The listing builds one solid part. Answer for the finished solid, in the listing's coordinates (mm). Face numbers are marked on the shaded views. A direction names the side the tool comes from. Coordinates: 2 decimals unless noted, no trailing zeros. Order: outer loops, then holes, each group sorted by start corner. A loop starts at its lowest first (then second) coordinate and runs counter-clockwise, first axis right, second up. Notation, with made-up numbers: (21.5, 64.25) - (35.5, 64.25) arc R11 ccw to (35.5, 81.25) - close; hole circle Ø3 at (30, 3.25). An arc over 180 degrees is marked (long way). Use one line per item in the form item = value. Start each with the question number.
Item 1: Section B-B, the plane z = 0 is taken. Write down the section's boundary in (x, y), and give its area (3 significant figures).
Item 2: Consider line 1 along X through (y, z) = (2.5, 0); line 2 along X through (y, z) = (5, 0); line 3 along Y through (x, z) = (7.5, 4). Determine where each line is inside the solid, lowest interval first. Write a range as [from, to].
Item 3: Each of these flat-tipped pins is pushed along its axis until it touches: pin 1 Ø4 at (y, z) = (17, -0.5) entering from -X; pin 2 Ø10 at (x, y) = (-20.5, 13) entering from +Z; pin 3 Ø8 at (y, z) = (28, 12.5) entering from -X. Where does it stop, or does it pass through?
Item 4: Section C-C, the plane y = 34.5 is taken. Write down the section's boundary in (x, z), and give its area (3 significant figures).
Item 5: A tool of negligible diameter and unlimited length cuts with its end or side. For the marked faces 1, 2 and 3, from which of +Z, -Z, +X, -X, +Y, -Y can it reach the whole face along a straight path? Write none if from no direction.
Item 6: Section A-A, the plane x = 0 is taken. Write down the section's boundary in (y, z).
Item 7: Section D-D, the plane y = 10.5 is taken. Write down the section's boundary in (x, z).
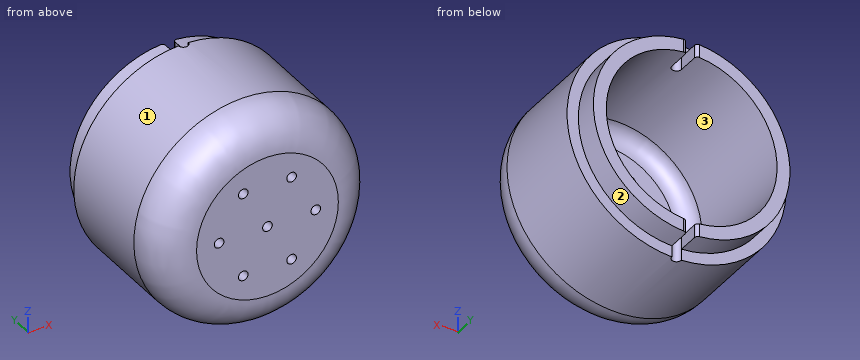
from build123d import *

# Parameters (mm, degrees)
ENL_V_MAT_EXTRU_1_REACH = 66.174
ESQUISSE2_R             = 1.5
ENL_V_MAT_EXTRU_2_DEPTH = 91.720725306
CONG_1_R                = 12
CONG_2_R                = 5
CONG_3_R                = 1


with BuildPart() as part:
    # Esquisse1 → Révolution1 (revolve)
    with BuildSketch(Plane(origin=(0, 0, 0), x_dir=(0, 0, -1), z_dir=(1, 0, 0)), mode=Mode.PRIVATE) as r_volution1_sk:
        Polygon((26.5, 49.5), (26.5, 7), (0, 7), (0, 0), (34, 0), (34, 42), (30.5, 42), (30.5, 49.5), align=None)
    revolve(r_volution1_sk.sketch.rotate(Axis((0, 7, 0), (0, -1, 0)), 180), axis=Axis((0, 7, 0), (0, -1, 0)))

    # Esquisse2 → Enlèv. mat.-Extru.1 (cut, up to next)
    with BuildSketch(Plane(origin=(0, 7, 0), x_dir=(1, 0, 0), z_dir=(0, 1, 0)), mode=Mode.PRIVATE) as enl_v_mat_extru_1_sk1:
        with Locations(Location((0, 0, 0), (0, 0, 270))):
            Circle(ESQUISSE2_R)
    enl_v_mat_extru_1_tool1 = extrude(enl_v_mat_extru_1_sk1.sketch, amount=-ENL_V_MAT_EXTRU_1_REACH, mode=Mode.PRIVATE) & part.part
    # Esquisse2 → Enlèv. mat.-Extru.1 (cut, up to next)
    with BuildSketch(Plane(origin=(0, 7, 0), x_dir=(1, 0, 0), z_dir=(0, 1, 0)), mode=Mode.PRIVATE) as enl_v_mat_extru_1_sk2:
        with Locations(Location((15, 0, 0), (0, 0, 270))):
            Circle(ESQUISSE2_R)
    enl_v_mat_extru_1_tool2 = extrude(enl_v_mat_extru_1_sk2.sketch, amount=-ENL_V_MAT_EXTRU_1_REACH, mode=Mode.PRIVATE) & part.part
    # Esquisse2 → Enlèv. mat.-Extru.1 (cut, up to next)
    with BuildSketch(Plane(origin=(0, 7, 0), x_dir=(1, 0, 0), z_dir=(0, 1, 0)), mode=Mode.PRIVATE) as enl_v_mat_extru_1_sk3:
        with Locations(Location((7.5, -12.990381057, 0), (0, 0, 270))):
            Circle(ESQUISSE2_R)
    enl_v_mat_extru_1_tool3 = extrude(enl_v_mat_extru_1_sk3.sketch, amount=-ENL_V_MAT_EXTRU_1_REACH, mode=Mode.PRIVATE) & part.part
    # Esquisse2 → Enlèv. mat.-Extru.1 (cut, up to next)
    with BuildSketch(Plane(origin=(0, 7, 0), x_dir=(1, 0, 0), z_dir=(0, 1, 0)), mode=Mode.PRIVATE) as enl_v_mat_extru_1_sk4:
        with Locations(Location((-7.5, -12.990381057, 0), (0, 0, 270))):
            Circle(ESQUISSE2_R)
    enl_v_mat_extru_1_tool4 = extrude(enl_v_mat_extru_1_sk4.sketch, amount=-ENL_V_MAT_EXTRU_1_REACH, mode=Mode.PRIVATE) & part.part
    # Esquisse2 → Enlèv. mat.-Extru.1 (cut, up to next)
    with BuildSketch(Plane(origin=(0, 7, 0), x_dir=(1, 0, 0), z_dir=(0, 1, 0)), mode=Mode.PRIVATE) as enl_v_mat_extru_1_sk5:
        with Locations(Location((-15, 0, 0), (0, 0, 270))):
            Circle(ESQUISSE2_R)
    enl_v_mat_extru_1_tool5 = extrude(enl_v_mat_extru_1_sk5.sketch, amount=-ENL_V_MAT_EXTRU_1_REACH, mode=Mode.PRIVATE) & part.part
    # Esquisse2 → Enlèv. mat.-Extru.1 (cut, up to next)
    with BuildSketch(Plane(origin=(0, 7, 0), x_dir=(1, 0, 0), z_dir=(0, 1, 0)), mode=Mode.PRIVATE) as enl_v_mat_extru_1_sk6:
        with Locations(Location((-7.5, 12.990381057, 0), (0, 0, 270))):
            Circle(ESQUISSE2_R)
    enl_v_mat_extru_1_tool6 = extrude(enl_v_mat_extru_1_sk6.sketch, amount=-ENL_V_MAT_EXTRU_1_REACH, mode=Mode.PRIVATE) & part.part
    # Esquisse2 → Enlèv. mat.-Extru.1 (cut, up to next)
    with BuildSketch(Plane(origin=(0, 7, 0), x_dir=(1, 0, 0), z_dir=(0, 1, 0)), mode=Mode.PRIVATE) as enl_v_mat_extru_1_sk7:
        with Locations(Location((7.5, 12.990381057, 0), (0, 0, 270))):
            Circle(ESQUISSE2_R)
    enl_v_mat_extru_1_tool7 = extrude(enl_v_mat_extru_1_sk7.sketch, amount=-ENL_V_MAT_EXTRU_1_REACH, mode=Mode.PRIVATE) & part.part
    add(enl_v_mat_extru_1_tool1.solids().sort_by_distance((0, 7, 0))[0], mode=Mode.SUBTRACT)
    add(enl_v_mat_extru_1_tool2.solids().sort_by_distance((15, 7, 0))[0], mode=Mode.SUBTRACT)
    add(enl_v_mat_extru_1_tool3.solids().sort_by_distance((7.5, 7, 12.990381))[0], mode=Mode.SUBTRACT)
    add(enl_v_mat_extru_1_tool4.solids().sort_by_distance((-7.5, 7, 12.990381))[0], mode=Mode.SUBTRACT)
    add(enl_v_mat_extru_1_tool5.solids().sort_by_distance((-15, 7, 0))[0], mode=Mode.SUBTRACT)
    add(enl_v_mat_extru_1_tool6.solids().sort_by_distance((-7.5, 7, -12.990381))[0], mode=Mode.SUBTRACT)
    add(enl_v_mat_extru_1_tool7.solids().sort_by_distance((7.5, 7, -12.990381))[0], mode=Mode.SUBTRACT)

    # Esquisse3 → Enlèv. mat.-Extru.2 (cut, through all)
    with BuildSketch(Plane.XY.offset(34)):
        with BuildLine():
            Line((-1.5, 42), (-1.5, 49.5))
            Line((-1.5, 49.5), (1.5, 49.5))
            Line((1.5, 49.5), (1.5, 42))
            ThreePointArc((1.5, 42), (0, 40.5), (-1.5, 42))
        make_face()
    extrude(amount=-ENL_V_MAT_EXTRU_2_DEPTH, mode=Mode.SUBTRACT)

    # Congé1
    cong_1_edges = [part.edges().sort_by_distance(p)[0] for p in [
        (0, 0, -34),
    ]]
    fillet(cong_1_edges, radius=CONG_1_R)

    # Congé2
    cong_2_edges = [part.edges().sort_by_distance(p)[0] for p in [
        (0, 7, -26.5),
    ]]
    fillet(cong_2_edges, radius=CONG_2_R)

    # Congé3
    cong_3_edges = [part.edges().sort_by_distance(p)[0] for p in [
        (-1.5, 49.5, -28.460302767),
        (-1.5, 49.5, 28.460302767),
        (1.5, 49.5, -28.460302767),
        (1.5, 49.5, 28.460302767),
    ]]
    fillet(cong_3_edges, radius=CONG_3_R)


solid = part.part
Response:
q1.outline = (-34, 12) arc R12 ccw to (-22, 0) - (-16.5, 0) - (-16.5, 7) - (-21.5, 7) arc R5 cw to (-26.5, 12) - (-26.5, 49.5) - (-30.5, 49.5) - (-30.5, 42) - (-34, 42) - close; (-13.5, 0) - (-1.5, 0) - (-1.5, 7) - (-13.5, 7) - close; (1.5, 0) - (13.5, 0) - (13.5, 7) - (1.5, 7) - close; (16.5, 0) - (22, 0) arc R12 ccw to (34, 12) - (34, 42) - (30.5, 42) - (30.5, 49.5) - (26.5, 49.5) - (26.5, 12) arc R5 cw to (21.5, 7) - (16.5, 7) - close
q1.area = 947 mm2
q2.line_1 = [-29.33, -16.5], [-13.5, -1.5], [1.5, 13.5], [16.5, 29.33]
q2.line_2 = [-31.75, -16.5], [-13.5, -1.5], [1.5, 13.5], [16.5, 31.75]
q2.line_3 = [0, 7]
q3.pin_1 = -34
q3.pin_2 = 30.26
q3.pin_3 = -32.92
q4.outline = circle Ø68 at (0, 0); hole circle Ø53 at (0, 0)
q4.area = 1,430 mm2
q5.face_1 = +Y, -Y
q5.face_2 = +X, +Y
q5.face_3 = +Y
q6.outline = (0, -22) arc R12 ccw to (12, -34) - (40.5, -34) - (40.5, -26.5) - (12, -26.5) arc R5 cw to (7, -21.5) - (7, -1.5) - (0, -1.5) - close; (0, 1.5) - (7, 1.5) - (7, 21.5) arc R5 cw to (12, 26.5) - (40.5, 26.5) - (40.5, 34) - (12, 34) arc R12 ccw to (0, 22) - close
q7.outline = circle Ø67.81 at (0, 0); hole circle Ø52.54 at (0, 0)
